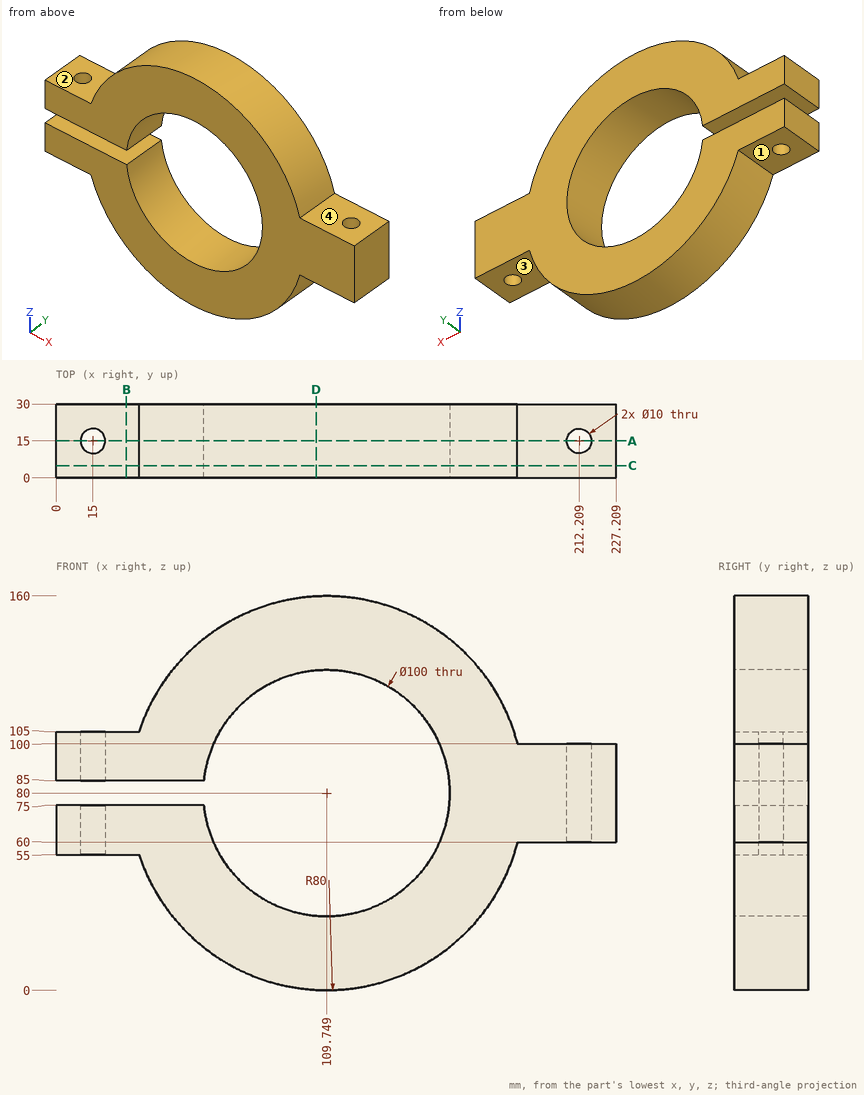
Part print with two shaded views. Sizes in mm from the minimum x, y, z corner. A direction names the side the tool comes from. Round coordinates to 2 decimals unless told otherwise and drop trailing zeros. Loops run counter-clockwise (first coordinate to the right, second up) from the corner with the lowest first, then second, coordinate; pieces in that order, holes last. Notation, with made-up numbers: M 0,-30 L 29,-30 A11 ccw 29,-21 Z; hole C -6.5,77.25 d8. An arc over 180 degrees is marked long. Put each result on its own line as item: value. Start each with the question number.
Item 1: Cut at C-C (y = 5). List the corners of the cut face in (x, z), then the cut area to 3 significant figures.
Item 2: 3-axis set-ups, long thin cutter, end or side, ignore diameter. For the marked faces 1, 2, 3 and 4: which of +Z, -Z, +X, -X, +Y, -Y reach the whole face in a straight line?
Item 3: Drop flat-ended pins along their axis: P1, Ø9, axis at x = 26.5, y = 18, coming from the +Z side; P2, Ø1.5, axis at x = 179.5, y = 22, coming from the +Z side (1 decimal); P3, Ø9, axis at x = 33.5, y = 9.5, coming from the -Z side (1 decimal); P4, Ø8, axis at x = 15, y = 15, coming from the +Z side. Give the stop position or say it passes through.
Item 4: Cut at B-B (x = 28.5). List the corners of the cut face in (y, z), then the cut area to 3 significant figures.
Item 5: Cut at A-A (y = 15). List the corners of the cut face in (x, z), then the cut area to 3 significant figures.
Item 6: Cut at D-D (x = 105.5). List the corners of the cut face in (y, z).
Item 7: Drill centre lines: line 1 along Y through (x, z) = (15, 96.25); line 2 along Z through (x, y) = (109.5, 25.5); line 3 along Z through (x, y) = (30, 26.25). Where is each one in solid material? Low to high.
Answer block:
1. outline: M 0,55 L 33.76,55 A80 ccw 187.21,60 L 227.21,60 L 227.21,100 L 187.21,100 A80 ccw 33.76,105 L 0,105 L 0,85 L 60,85 A50 cw long 60,75 L 0,75 Z
1. area: 14,700 mm2
2. face 1: -Z, -X, +Y, -Y
2. face 2: +Z, -X, +Y, -Y
2. face 3: -Z, +X, +Y, -Y
2. face 4: +Z, +X, +Y, -Y
3. P1: z = 105
3. P2: z = 120.5
3. P3: z = 44.6
3. P4: through
4. outline: M 0,55 L 30,55 L 30,75 L 0,75 Z; M 0,85 L 30,85 L 30,105 L 0,105 Z
4. area: 1,200 mm2
5. outline: M 0,55 L 10,55 L 10,75 L 0,75 Z; M 0,85 L 10,85 L 10,105 L 0,105 Z; M 20,55 L 33.76,55 A80 ccw 187.21,60 L 207.21,60 L 207.21,100 L 187.21,100 A80 ccw 33.76,105 L 20,105 L 20,85 L 60,85 A50 cw long 60,75 L 20,75 Z; M 217.21,60 L 227.21,60 L 227.21,100 L 217.21,100 Z
5. area: 13,900 mm2
6. outline: M 0,0.11 L 30,0.11 L 30,30.18 L 0,30.18 Z; M 0,129.82 L 30,129.82 L 30,159.89 L 0,159.89 Z
7. line 1: 0 to 10, 20 to 30
7. line 2: 0 to 30, 130 to 160
7. line 3: 55 to 75, 85 to 105
